```python
from build123d import *

# Parameters (mm, degrees)
F1_R     = 125
F1_R_2   = 15
F2_DEPTH = 10
F3_R     = 8
F4_SIZE  = 5
F5_R     = 10.046547
F6_DEPTH = 250
F7_DEPTH = 250


with BuildPart() as f2:
    # F1 (on face) → F2 (new body)
    with BuildSketch(Plane.XY):
        Circle(F1_R)
        with Locations((-48.868799, -40.720446)):
            Circle(F1_R_2, mode=Mode.SUBTRACT)
        with Locations((-0.93582, -60.962566)):
            Circle(F1_R_2, mode=Mode.SUBTRACT)
        with Locations((47.271254, -41.382171)):
            Circle(F1_R_2, mode=Mode.SUBTRACT)
        with Locations((-68.449193, 7.486627)):
            Circle(F1_R_2, mode=Mode.SUBTRACT)
        with Locations((-48.207074, 55.419606)):
            Circle(F1_R_2, mode=Mode.SUBTRACT)
        with Locations((47.932978, 54.757881)):
            Circle(F1_R_2, mode=Mode.SUBTRACT)
        with Locations((67.513373, 6.550807)):
            Circle(F1_R_2, mode=Mode.SUBTRACT)
        with Locations((0, 75)):
            Circle(F1_R_2, mode=Mode.SUBTRACT)
    extrude(amount=F2_DEPTH)

    # F3
    f3_edges = [f2.edges().sort_by_distance(p)[0] for p in [
        (-125, 0, 10),
    ]]
    fillet(f3_edges, radius=F3_R)

    # F4
    f4_edges = [f2.edges().sort_by_distance(p)[0] for p in [
        (-15.93582, -60.962566, 10),
    ]]
    chamfer(f4_edges, length=F4_SIZE)

    # F5 (on face) → F6 (join)
    with BuildSketch(Plane.XY):
        with Locations((52.640375, -21.991979)):
            Circle(F5_R)
    extrude(amount=-F6_DEPTH)

    # F5 (on face) → F7 (join)
    with BuildSketch(Plane.XY):
        with Locations((-21.991979, -52.640375)):
            Circle(F5_R)
        with Locations((52.640375, -21.991979)):
            Circle(F5_R)
        with Locations((21.991979, 52.640375)):
            Circle(F5_R)
        with Locations((-52.640375, 21.991979)):
            Circle(F5_R)
    extrude(amount=-F7_DEPTH)


solid = f2.part
```
Geometry: final body of the model. Coordinates: model frame, mm. A direction names the side the tool comes from. Round coordinates to 2 decimals unless told otherwise and drop trailing zeros. Order: outer loops, then holes, each group sorted by start corner. A loop starts at its lowest first (then second) coordinate and runs counter-clockwise, first axis right, second up. Notation, with made-up numbers: (21.25, 43) -> (37.25, 43) arc R23 ccw to (37.25, 79) -> close; hole circle Ø11 at (84.5, 67). An arc over 180 degrees is marked (long way). Use one line per item in the form item = value.
(1) Section C-C on z = -216.5. Return loops of the section in (x, y).
Results list:
outline = circle Ø20.09 at (-52.64, 21.99); circle Ø20.09 at (-21.99, -52.64); circle Ø20.09 at (21.99, 52.64); circle Ø20.09 at (52.64, -21.99)
(2) First-contact query: pin 1 Ø2 at (y, z) = (12.5, -107) entering from -X; pin 2 Ø12 at (x, z) = (16.5, -170.5) entering from +Y; pin 3 Ø3 at (x, z) = (-34.5, -81.5) entering from +Y; pin 4 Ø1.7 at (x, y) = (50, -30.5) entering from +Z. Flat tips, straight axial feed; report the tip coordinate or a pass-through.
Results list:
pin_1 = -58.01
pin_2 = 62.69
pin_3 = through
pin_4 = 0
(3) Access query for faces 5 (the face through (52, -22, -250)), 6 (the face through (42.6, -21.6, -123.2)), 7 (the face through (61.127, -47.127, 4.93)). Directions: +Z, -Z, +X, -X, +Y, -Y. A direction counts if a zero-diameter tool reaches every point of the face in a straight line with its end or side. Return the directions, or none.
Results list:
face_5 = -Z, +X, -X, +Y, -Y
face_6 = -Z
face_7 = +Z
(4) Ray query, probe 1 along Y at (x, z) = (-52.5, -10.5); probe 2 along Z at (x, y) = (-17, 24); probe 3 along Y at (x, z) = (21.5, -79). Return the intervals inside material, ascending. Write a range as [from, to].
Results list:
probe_1 = [11.95, 32.04]
probe_2 = [0, 10]
probe_3 = [42.61, 62.67]
(5) Section A-A on y = 0. Return loops of the section in (x, z), and give its area (3 significant figures).
Results list:
outline = (-125, 0) -> (-81.45, 0) -> (-81.45, 10) -> (-117, 10) arc R8 ccw to (-125, 2) -> close; (-55.45, 0) -> (54.02, 0) -> (54.02, 10) -> (-55.45, 10) -> close; (81.01, 0) -> (125, 0) -> (125, 2) arc R8 ccw to (117, 10) -> (81.01, 10) -> close
area = 1,940 mm^2
(6) Section B-B on x = 3. Count the separate pieces of the cut face and the enclosed holes in it, and give its area (3 significant figures).
Results list:
separate_pieces = 3
enclosed_holes = 0
area = 1,860 mm^2
(7) Draft query along Y for faces 1 (the face through (-2, 2, 10)), 2 (the face through (31.27, 48.79, -123.25)), 3 (the face through (-79.505, 17.624, 4.93)), 4 (the face through (-58, 17, 0)). Return one class per face: pulls with the +Y half, pulls with the -Y half, needs draft (parallel to the pull), parting line crosses it, or undercut.
Results list:
face_1 = needs draft
face_2 = parting line crosses it
face_3 = undercut
face_4 = undercut
